Here's how the part is built. I have some questions about the finished solid (model axes, mm). Face numbers are marked on the shaded views. Round coordinates to 2 decimals unless told otherwise and drop trailing zeros. Loops run counter-clockwise (first coordinate to the right, second up) from the corner with the lowest first, then second, coordinate; pieces in that order, holes last. Notation, with made-up numbers: M -9,-5.75 L 0,-5.75 A14 cw 0,-0.75 Z; hole C 21.25,-11 d9. An arc over 180 degrees is marked long. Use a Markdown table: item, result.
```python
from build123d import *

# Parameters (mm, degrees)
F1_DEPTH = 3
F2_R     = 50
F3_W     = 1400
F3_H     = 40
F4_DEPTH = 40


with BuildPart() as f1:
    # F0 (on Front) → F1 (new body)
    with BuildSketch(Plane.XZ):
        with BuildLine():
            Line((80, 503.1805617435), (-80, 474.9682448302))
            Line((-80, 474.9682448302), (-80, 400))
            ThreePointArc((-80, 400), (-182.5126265847, 152.5126265847), (-430, 50))
            Line((-430, 50), (-700, 50))
            Line((-700, 50), (-700, 0))
            Line((-700, 0), (700, 0))
            Line((700, 0), (700, 50))
            Line((700, 50), (430, 50))
            ThreePointArc((430, 50), (182.5126265847, 152.5126265847), (80, 400))
            Line((80, 400), (80, 503.1805617435))
        make_face()
        with BuildLine():
            Line((-881.9857732693, 369.0964462745), (-492.5372057432, 437.7667363276))
            ThreePointArc((-492.5372057432, 437.7667363276), (-502.2519540362, 461.4394293899), (-501.2196146265, 487.0071239782))
            Line((-501.2196146265, 487.0071239782), (-890.6681821527, 418.3368339251))
            Line((-890.6681821527, 418.3368339251), (-881.9857732693, 369.0964462745))
        make_face()
        with BuildLine():
            Line((-438.8222844138, 447.2381262246), (-443.1634888555, 471.8583200499))
            Line((-443.1634888555, 471.8583200499), (-447.5046932972, 496.4785138752))
            Line((-447.5046932972, 496.4785138752), (-501.2196146265, 487.0071239782))
            ThreePointArc((-501.2196146265, 487.0071239782), (-502.2519540362, 461.4394293899), (-492.5372057432, 437.7667363276))
            Line((-492.5372057432, 437.7667363276), (-438.8222844138, 447.2381262246))
        make_face()
        with BuildLine():
            ThreePointArc((-383.1634888555, 471.8583200499), (-383.39180697, 477.0876646147), (-384.0750236748, 482.2772107099))
            Line((-384.0750236748, 482.2772107099), (-443.1634888555, 471.8583200499))
            Line((-443.1634888555, 471.8583200499), (-438.8222844138, 447.2381262246))
            Line((-438.8222844138, 447.2381262246), (-385.1073630845, 456.7095161216))
            ThreePointArc((-385.1073630845, 456.7095161216), (-383.6514415614, 464.2218138547), (-383.1634888555, 471.8583200499))
        make_face()
        with BuildLine():
            Line((-443.1634888555, 471.8583200499), (-384.0750236748, 482.2772107099))
            ThreePointArc((-384.0750236748, 482.2772107099), (-387.6557386402, 494.6374698592), (-393.7897719678, 505.9499037722))
            Line((-393.7897719678, 505.9499037722), (-447.5046932972, 496.4785138752))
            Line((-447.5046932972, 496.4785138752), (-443.1634888555, 471.8583200499))
        make_face()
        with BuildLine():
            Line((-393.7897719678, 505.9499037722), (-4.3412044417, 574.6201938253))
            Line((-4.3412044417, 574.6201938253), (-10.41889066, 609.0884651807))
            Line((-10.41889066, 609.0884651807), (-453.5823795155, 530.9467852306))
            ThreePointArc((-453.5823795155, 530.9467852306), (-420.0208735696, 527.2155179354), (-393.7897719678, 505.9499037722))
        make_face()
        with BuildLine():
            Line((-80, 535.8938415433), (-80, 550))
            Line((-80, 550), (0, 550))
            Line((0, 550), (-4.3412044417, 574.6201938253))
            Line((-4.3412044417, 574.6201938253), (-393.7897719678, 505.9499037722))
            ThreePointArc((-393.7897719678, 505.9499037722), (-387.6557386402, 494.6374698592), (-384.0750236748, 482.2772107099))
            Line((-384.0750236748, 482.2772107099), (-80, 535.8938415433))
        make_face()
        with BuildLine():
            Line((-80, 510.5081762462), (-80, 535.8938415433))
            Line((-80, 535.8938415433), (-384.0750236748, 482.2772107099))
            ThreePointArc((-384.0750236748, 482.2772107099), (-383.39180697, 477.0876646147), (-383.1634888555, 471.8583200499))
            ThreePointArc((-383.1634888555, 471.8583200499), (-383.6514415614, 464.2218138547), (-385.1073630845, 456.7095161216))
            Line((-385.1073630845, 456.7095161216), (-80, 510.5081762462))
        make_face()
        with BuildLine():
            Line((-80, 474.9682448302), (-80, 510.5081762462))
            Line((-80, 510.5081762462), (-385.1073630845, 456.7095161216))
            ThreePointArc((-385.1073630845, 456.7095161216), (-402.4832672908, 427.7548102865), (-432.7445981955, 412.7698548691))
            Line((-432.7445981955, 412.7698548691), (-80, 474.9682448302))
        make_face()
        Polygon((80, 538.7204931595), (-80, 510.5081762462), (-80, 474.9682448302), (80, 503.1805617435), align=None)
        Polygon((0, 550), (-80, 535.8938415433), (-80, 510.5081762462), (80, 538.7204931595), (80, 550), align=None)
        Polygon((0, 550), (-80, 550), (-80, 535.8938415433), align=None)
        with BuildLine():
            Line((443.1634888555, 628.1416799501), (384.0750236748, 617.7227892901))
            ThreePointArc((384.0750236748, 617.7227892901), (387.6557386402, 605.3625301408), (393.7897719678, 594.0500962278))
            Line((393.7897719678, 594.0500962278), (447.5046932972, 603.5214861248))
            Line((447.5046932972, 603.5214861248), (443.1634888555, 628.1416799501))
        make_face()
        with BuildLine():
            Line((-4.3412044417, 574.6201938253), (0, 550))
            Line((0, 550), (384.0750236748, 617.7227892901))
            ThreePointArc((384.0750236748, 617.7227892901), (383.2123374991, 630.5623102494), (385.1073630845, 643.2904838784))
            Line((385.1073630845, 643.2904838784), (-4.3412044417, 574.6201938253))
        make_face()
        with BuildLine():
            Line((447.5046932972, 603.5214861248), (393.7897719678, 594.0500962278))
            ThreePointArc((393.7897719678, 594.0500962278), (420.0208735696, 572.7844820646), (453.5823795155, 569.0532147694))
            Line((453.5823795155, 569.0532147694), (447.5046932972, 603.5214861248))
        make_face()
        with BuildLine():
            ThreePointArc((432.7445981955, 687.2301451309), (402.4832672908, 672.2451897135), (385.1073630845, 643.2904838784))
            Line((385.1073630845, 643.2904838784), (438.8222844138, 652.7618737754))
            Line((438.8222844138, 652.7618737754), (432.7445981955, 687.2301451309))
        make_face()
        with BuildLine():
            Line((393.7897719678, 594.0500962278), (80, 538.7204931595))
            Line((80, 538.7204931595), (80, 503.1805617435))
            Line((80, 503.1805617435), (453.5823795155, 569.0532147694))
            ThreePointArc((453.5823795155, 569.0532147694), (420.0208735696, 572.7844820646), (393.7897719678, 594.0500962278))
        make_face()
        with BuildLine():
            ThreePointArc((385.1073630845, 643.2904838784), (383.2123374991, 630.5623102494), (384.0750236748, 617.7227892901))
            Line((384.0750236748, 617.7227892901), (443.1634888555, 628.1416799501))
            Line((443.1634888555, 628.1416799501), (438.8222844138, 652.7618737754))
            Line((438.8222844138, 652.7618737754), (385.1073630845, 643.2904838784))
        make_face()
        with BuildLine():
            Line((384.0750236748, 617.7227892901), (0, 550))
            Line((0, 550), (80, 550))
            Line((80, 550), (80, 538.7204931595))
            Line((80, 538.7204931595), (393.7897719678, 594.0500962278))
            ThreePointArc((393.7897719678, 594.0500962278), (387.6557386402, 605.3625301408), (384.0750236748, 617.7227892901))
        make_face()
        with BuildLine():
            Line((-10.41889066, 609.0884651807), (-4.3412044417, 574.6201938253))
            Line((-4.3412044417, 574.6201938253), (385.1073630845, 643.2904838784))
            ThreePointArc((385.1073630845, 643.2904838784), (402.4832672908, 672.2451897135), (432.7445981955, 687.2301451309))
            Line((432.7445981955, 687.2301451309), (-10.41889066, 609.0884651807))
        make_face()
        with BuildLine():
            Line((881.9857732693, 730.9035537255), (492.5372057432, 662.2332636724))
            ThreePointArc((492.5372057432, 662.2332636724), (500.4453490438, 645.9963290189), (503.1634888555, 628.1416799501))
            ThreePointArc((503.1634888555, 628.1416799501), (502.6755361496, 620.5051737549), (501.2196146265, 612.9928760218))
            Line((501.2196146265, 612.9928760218), (890.6681821527, 681.6631660749))
            Line((890.6681821527, 681.6631660749), (881.9857732693, 730.9035537255))
        make_face()
        with BuildLine():
            Line((438.8222844138, 652.7618737754), (443.1634888555, 628.1416799501))
            Line((443.1634888555, 628.1416799501), (447.5046932972, 603.5214861248))
            Line((447.5046932972, 603.5214861248), (501.2196146265, 612.9928760218))
            ThreePointArc((501.2196146265, 612.9928760218), (502.6755361496, 620.5051737549), (503.1634888555, 628.1416799501))
            ThreePointArc((503.1634888555, 628.1416799501), (500.4453490438, 645.9963290189), (492.5372057432, 662.2332636724))
            Line((492.5372057432, 662.2332636724), (438.8222844138, 652.7618737754))
        make_face()
        with BuildLine():
            Line((-447.5046932972, 496.4785138752), (-393.7897719678, 505.9499037722))
            ThreePointArc((-393.7897719678, 505.9499037722), (-420.0208735696, 527.2155179354), (-453.5823795155, 530.9467852306))
            Line((-453.5823795155, 530.9467852306), (-447.5046932972, 496.4785138752))
        make_face()
        with BuildLine():
            ThreePointArc((-432.7445981955, 412.7698548691), (-402.4832672908, 427.7548102865), (-385.1073630845, 456.7095161216))
            Line((-385.1073630845, 456.7095161216), (-438.8222844138, 447.2381262246))
            Line((-438.8222844138, 447.2381262246), (-432.7445981955, 412.7698548691))
        make_face()
    extrude(amount=F1_DEPTH)

    # F2
    f2_edges = [f1.edges().sort_by_distance(p)[0] for p in [
        (-80, -1.5, 474.968245),
        (80, -1.5, 503.180562),
    ]]
    fillet(f2_edges, radius=F2_R)

    # F3 (on face) → F4 (join)
    with BuildSketch(Plane.XZ):
        with Locations((0, 20)):
            Rectangle(F3_W, F3_H)
    extrude(amount=-F4_DEPTH)


solid = f1.part
```
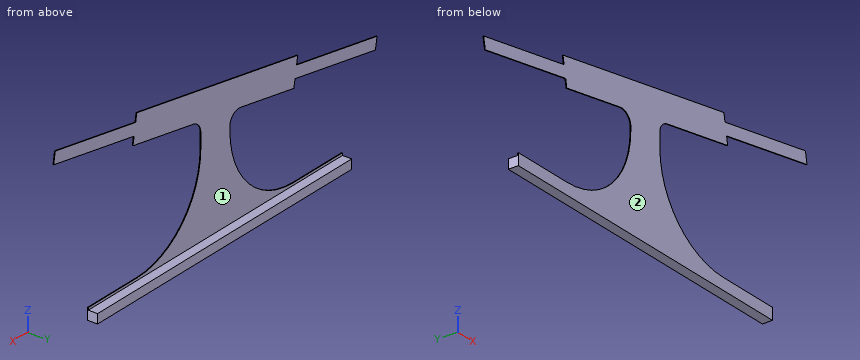
Q1. Imagine slicing it at A-A, the plane x = -114.5. Please give me the cut outline in (y, z).
Return value:
| item | result |
|---|---|
| outline | M -3,0 L 40,0 L 40,40 L 0,40 L 0,248.48 L -3,248.48 Z; M -3,462.92 L 0,462.92 L 0,590.74 L -3,590.74 Z |
Q2. Imagine slicing it at D-D, the plane z = 185. Please give me the cut outline in (x, y).
Return value:
| item | result |
|---|---|
| outline | M -153.82,-3 L 153.82,-3 L 153.82,0 L -153.82,0 Z |
Q3. Will these pins go through, and if not, where does the flat tip stop? P1, Ø0.9, axis at y = -1, z = 443, coming from the +X side; P2, Ø1, axis at x = 282.5, y = 35, coming from the +Z side; P3, Ø0.9, axis at x = 555.5, y = -1.5, coming from the +Z side.
Return value:
| item | result |
|---|---|
| P1 | stops at x = 80 |
| P2 | stops at z = 40 |
| P3 | stops at z = 673.41 |
Q4. I need wall thicknesses on line 1 (Y direction, x = -18, z = 44); line 2 (Z direction, x = -663.5, y = 1); line 3 (X direction, y = 33, z = 36). Which ranges of each line are inside material? Lowest first, please. Write a range as from..to.
Return value:
| item | result |
|---|---|
| line 1 | y = -3..0 |
| line 2 | z = 0..40 |
| line 3 | x = -700..700 |
Q5. We'd pull the mould along Y, two halves only. Please class the marked faces 1 and 2: pulls with the +Y half, pulls with the -Y half, needs draft (parallel to the pull), parting line crosses it, or undercut.
Return value:
| item | result |
|---|---|
| face 1 | pulls with the +Y half |
| face 2 | pulls with the -Y half |
Q6. Imagine slicing it at C-C, the plane x = 585.5. Please give me the cut outline in (y, z), then the cut area to 3 significant figures.
Return value:
| item | result |
|---|---|
| outline | M -3,0 L 40,0 L 40,40 L 0,40 L 0,50 L -3,50 Z; M -3,627.85 L 0,627.85 L 0,678.63 L -3,678.63 Z |
| area | 1,900 mm^2 |
Q7. Imagine slicing it at B-B, the plane y = 21.5. Please give me the cut outline in (x, z).
Return value:
| item | result |
|---|---|
| outline | M -700,0 L 700,0 L 700,40 L -700,40 Z |
